Model file for the job. Use its own axes, mm. A direction names the side the tool comes from. Coordinates: 2 decimals unless noted, no trailing zeros. Order: outer loops, then holes, each group sorted by start corner. A loop starts at its lowest first (then second) coordinate and runs counter-clockwise, first axis right, second up.
from build123d import *

# Parameters (mm, degrees)
SKETCH1_W           = 70
SKETCH1_H           = 70
BOSS_EXTRUDE1_DEPTH = 15
SKETCH2_R           = 30
SKETCH2_R_2         = 25
SKETCH2_R_3         = 3.5
CUT_EXTRUDE1_DEPTH  = 5
SKETCH3_R           = 3.5
CUT_EXTRUDE2_DEPTH  = 16
SKETCH4_R           = 10
CUT_EXTRUDE3_DEPTH  = 16


with BuildPart() as part:
    # Sketch1 → Boss-Extrude1 (new body)
    with BuildSketch(Plane.XY):
        Rectangle(SKETCH1_W, SKETCH1_H)
    extrude(amount=BOSS_EXTRUDE1_DEPTH)

    # Sketch2 → Cut-Extrude1 (cut)
    with BuildSketch(Plane.XY.offset(15)):
        Circle(SKETCH2_R)
        Circle(SKETCH2_R_2, mode=Mode.SUBTRACT)
        with Locations((-25.229863316, 27.137958195)):
            Circle(SKETCH2_R_3)
        with Locations((25.229863316, 27.137958195)):
            Circle(SKETCH2_R_3)
        with Locations((25.229863316, -27.137958195)):
            Circle(SKETCH2_R_3)
        with Locations((-25.229863316, -27.137958195)):
            Circle(SKETCH2_R_3)
    extrude(amount=-CUT_EXTRUDE1_DEPTH, mode=Mode.SUBTRACT)

    # Sketch3 → Cut-Extrude2 (cut, through all)
    with BuildSketch(Plane.XY):
        with Locations((-25.229863316, 27.137958195)):
            Circle(SKETCH3_R)
        with Locations((25.229863316, 27.137958195)):
            Circle(SKETCH3_R)
        with Locations((25.229863316, -27.137958195)):
            Circle(SKETCH3_R)
        with Locations((-25.229863316, -27.137958195)):
            Circle(SKETCH3_R)
    extrude(amount=CUT_EXTRUDE2_DEPTH, mode=Mode.SUBTRACT)

    # Sketch4 → Cut-Extrude3 (cut, through all)
    with BuildSketch(Plane(origin=(0, 0, 0), x_dir=(-1, 0, 0), z_dir=(0, 0, -1))):
        Circle(SKETCH4_R)
    extrude(amount=-CUT_EXTRUDE3_DEPTH, mode=Mode.SUBTRACT)


solid = part.part
Q1. Cut at C-C, the plane z = 5.75. List the corners of the cut face in (x, y), plus the area to 3 significant figures.
Established:
outline: (-35, -35) - (35, -35) - (35, 35) - (-35, 35) - close; hole circle Ø7 at (-25.23, -27.14); hole circle Ø7 at (-25.23, 27.14); hole circle Ø20 at (0, 0); hole circle Ø7 at (25.23, -27.14); hole circle Ø7 at (25.23, 27.14)
area: 4,430 mm2
Q2. Mould opens along X. For faces 3 (the face through (-7, 25, 10)), 4 (the face through (35, 0, 7)), 5 (the face through (0, -11, 15)) say: pulls with the +X half, pulls with the -X half, needs draft (parallel to the pull), parting line crosses it, or undercut.
Established:
face 3: undercut
face 4: pulls with the +X half
face 5: needs draft
Q3. Cut at A-A, the plane y = 0. List the corners of the cut face in (x, z), plus the area to 3 significant figures.
Established:
outline: (-35, 0) - (-10, 0) - (-10, 15) - (-25, 15) - (-25, 10) - (-30, 10) - (-30, 15) - (-35, 15) - close; (10, 0) - (35, 0) - (35, 15) - (30, 15) - (30, 10) - (25, 10) - (25, 15) - (10, 15) - close
area: 700 mm2
Q4. Cut at D-D, the plane x = 15.5. List the corners of the cut face in (y, z).
Established:
outline: (-35, 0) - (35, 0) - (35, 15) - (25.69, 15) - (25.69, 10) - (19.62, 10) - (19.62, 15) - (-19.62, 15) - (-19.62, 10) - (-25.69, 10) - (-25.69, 15) - (-35, 15) - close
Q5. Probe line 1 (X direction, y = -27, z = 2); line 2 (Y direction, x = 0, z = 13.55); line 3 (X direction, y = -12, z = 11.5). List the from-to ranges inside material, lowest first.
Established:
line 1: x = -35 to -28.73, -21.73 to 21.73, 28.73 to 35
line 2: y = -35 to -30, -25 to -10, 10 to 25, 30 to 35
line 3: x = -35 to -27.5, -21.93 to 21.93, 27.5 to 35
Q6. Which spindle directions (+Z, -Z, +X, -X, +Y, -Y) get a long thin tool onto all of the face, cutting with end or side? Do faces 1 (the face through (-29.97, 1.32, 12.54)), 2 (the face through (-27.81, 29.5, 7.4)). Say none if no direction does.
Established:
face 1: +Z
face 2: +Z, -Z
